The model under review builds one solid part; all positions refer to its coordinate system, in mm. A direction names the side the tool comes from. Give positions to 0.01 mm unless a question says otherwise; leave off trailing zeros. Order: outer loops, then holes, each group sorted by start corner. A loop starts at its lowest first (then second) coordinate and runs counter-clockwise, first axis right, second up. Notation, with made-up numbers: (-16.75, 77.5) - (25.25, 77.5) arc R30 ccw to (25.25, 116.5) - close; hole circle Ø3 at (4, 29.25). An arc over 180 degrees is marked (long way). Use a Markdown table: item, result. Add a question column.
```python
from build123d import *

# Parameters (mm, degrees)
F1_DEPTH  = 12.7
F2_R      = 7.5104207728
F3_DEPTH  = 12.701
F4_W      = 187.1625185013
F4_H      = 16.4809370326
F4_W_2    = 34.8658077419
F4_H_2    = 35.9553694725
F5_DEPTH  = 12.7
F5_FACE_R = 7.5104207728
F5_FACE_W = 34.8658077419
F5_FACE_H = 35.9553694725
F6_DEPTH  = 25.4
F7_DEPTH  = 12.7
F9_DEPTH  = 38.354


with BuildPart() as f1:
    # F0 (on Top) → F1 (new body)
    with BuildSketch(Plane.XY):
        Polygon((21.6443181937, 44.9448898435), (-21.6443181937, 44.9448898435), (-48.6343415176, 11.1004710827), (-39.001713719, -31.1028288117), (0, -49.8850642288), (39.001713719, -31.1028288117), (48.6343415176, 11.1004710827), align=None)
    extrude(amount=F1_DEPTH)

    # F2 (on face) → F3 (cut, through all)
    with BuildSketch(Plane.XY.offset(12.7)):
        with Locations((-21.6443181937, 11.1004710827)):
            Circle(F2_R)
        with Locations((21.6443181937, 11.1004710827)):
            Circle(F2_R)
        with BuildLine():
            ThreePointArc((-22.3923972439, -17.5961239861), (-20.1468702335, -19.4861496183), (-17.2912654826, -20.1644636691))
            Line((-17.2912654826, -20.1644636691), (19.5472728087, -20.1644636691))
            ThreePointArc((19.5472728087, -20.1644636691), (21.5385429204, -19.8441687483), (23.3289331258, -18.9155954304))
            Line((23.3289331258, -18.9155954304), (29.0724616498, -14.657702297))
            Line((29.0724616498, -14.657702297), (-24.5707594616, -14.657702297))
            Line((-24.5707594616, -14.657702297), (-22.3923972439, -17.5961239861))
        make_face()
    extrude(amount=-F3_DEPTH, mode=Mode.SUBTRACT)

    # F4 (on face) → F5 (join)
    with BuildSketch(Plane.XY.offset(12.7)):
        with BuildLine():
            Line((56.5410580551, -83.4953508641), (19.5008568595, -74.5715907042))
            Line((19.5008568595, -74.5715907042), (-19.5008568595, -74.5715907042))
            Line((-19.5008568595, -74.5715907042), (-56.5410580551, -83.4953508641))
            add(Edge.make_bspline(
                [(-56.5410580551, -83.4953508641), (-37.4583826818, -107.754176934), (0, -155.2743553327), (37.4583826818, -107.754176934), (56.5410580551, -83.4953508641)],
                knots=[0, 0, 0, 0, 0.5, 1, 1, 1, 1], degree=3))
        make_face()
        with BuildLine():
            Line((93.5812592506, -92.419111024), (56.5410580551, -83.4953508641))
            add(Edge.make_bspline(
                [(-56.5410580551, -83.4953508641), (-37.4583826818, -107.754176934), (0, -155.2743553327), (37.4583826818, -107.754176934), (56.5410580551, -83.4953508641)],
                knots=[0, 0, 0, 0, 0.5, 1, 1, 1, 1], degree=3))
            Line((-56.5410580551, -83.4953508641), (-93.5812592506, -92.419111024))
            Line((-93.5812592506, -92.419111024), (-93.5812592506, -135.6894243062))
            Line((-93.5812592506, -135.6894243062), (-93.5812592506, -239.1290962696))
            Line((-93.5812592506, -239.1290962696), (93.5812592506, -239.1290962696))
            Line((93.5812592506, -239.1290962696), (93.5812592506, -135.6894243062))
            Line((93.5812592506, -135.6894243062), (93.5812592506, -92.419111024))
        make_face()
        with BuildLine():
            Line((192.9354845729, -199.789452925), (93.5812592506, -92.419111024))
            Line((93.5812592506, -92.419111024), (93.5812592506, -135.6894243062))
            Line((93.5812592506, -135.6894243062), (171.3652932207, -219.7492445575))
            ThreePointArc((171.3652932207, -219.7492445575), (193.3684597033, -221.8925180787), (192.9354845729, -199.789452925))
        make_face()
        with BuildLine():
            Line((-93.5812592506, -135.6894243062), (-93.5812592506, -92.419111024))
            Line((-93.5812592506, -92.419111024), (-192.9354845729, -199.789452925))
            ThreePointArc((-192.9354845729, -199.789452925), (-193.3684597033, -221.8925180787), (-171.3652932207, -219.7492445575))
            Line((-171.3652932207, -219.7492445575), (-93.5812592506, -135.6894243062))
        make_face()
        with Locations((0, -247.3695647859)):
            Rectangle(F4_W, F4_H)
        Polygon((93.5812592506, -410.4407429695), (93.5812592506, -255.6100333022), (-93.5812592506, -255.6100333022), (-93.5812592506, -410.4407429695), (-67.6731318235, -410.4407429695), (-32.8073054552, -410.4407429695), (0, -410.4407429695), (32.8073054552, -410.4407429695), (67.6731318235, -410.4407429695), align=None)
        with Locations((57.6258767396, -294.4029867649)):
            Rectangle(F4_W_2, F4_H_2, mode=Mode.SUBTRACT)
        with BuildLine():
            Line((67.6731318235, -537.919596071), (67.6731318235, -410.4407429695))
            Line((67.6731318235, -410.4407429695), (32.8073054552, -410.4407429695))
            Line((32.8073054552, -410.4407429695), (32.8073054552, -537.919596071))
            ThreePointArc((32.8073054552, -537.919596071), (50.2402186394, -556.4753226857), (67.6731318235, -537.919596071))
        make_face()
        with BuildLine():
            Line((-32.8073054552, -410.4407429695), (-67.6731318235, -410.4407429695))
            Line((-67.6731318235, -410.4407429695), (-67.6731318235, -537.919596071))
            ThreePointArc((-67.6731318235, -537.919596071), (-50.2402186394, -556.4753226857), (-32.8073054552, -537.919596071))
            Line((-32.8073054552, -537.919596071), (-32.8073054552, -410.4407429695))
        make_face()
        Polygon((0, -49.8850642288), (-19.5008568595, -40.4939465203), (-19.5008568595, -74.5715907042), (19.5008568595, -74.5715907042), (19.5008568595, -40.4939465203), align=None)
    extrude(amount=-F5_DEPTH)

    # F4 (on face) + F5_face (on face) → F6 (join)
    with BuildSketch(Plane.XY.offset(12.7)):
        with BuildLine():
            Line((56.5410580551, -83.4953508641), (19.5008568595, -74.5715907042))
            Line((19.5008568595, -74.5715907042), (-19.5008568595, -74.5715907042))
            Line((-19.5008568595, -74.5715907042), (-56.5410580551, -83.4953508641))
            add(Edge.make_bspline(
                [(-56.5410580551, -83.4953508641), (-37.4583826818, -107.754176934), (0, -155.2743553327), (37.4583826818, -107.754176934), (56.5410580551, -83.4953508641)],
                knots=[0, 0, 0, 0, 0.5, 1, 1, 1, 1], degree=3))
        make_face()
        with BuildLine():
            Line((93.5812592506, -92.419111024), (56.5410580551, -83.4953508641))
            add(Edge.make_bspline(
                [(-56.5410580551, -83.4953508641), (-37.4583826818, -107.754176934), (0, -155.2743553327), (37.4583826818, -107.754176934), (56.5410580551, -83.4953508641)],
                knots=[0, 0, 0, 0, 0.5, 1, 1, 1, 1], degree=3))
            Line((-56.5410580551, -83.4953508641), (-93.5812592506, -92.419111024))
            Line((-93.5812592506, -92.419111024), (-93.5812592506, -135.6894243062))
            Line((-93.5812592506, -135.6894243062), (-93.5812592506, -239.1290962696))
            Line((-93.5812592506, -239.1290962696), (93.5812592506, -239.1290962696))
            Line((93.5812592506, -239.1290962696), (93.5812592506, -135.6894243062))
            Line((93.5812592506, -135.6894243062), (93.5812592506, -92.419111024))
        make_face()
        with BuildLine():
            Line((192.9354845729, -199.789452925), (93.5812592506, -92.419111024))
            Line((93.5812592506, -92.419111024), (93.5812592506, -135.6894243062))
            Line((93.5812592506, -135.6894243062), (171.3652932207, -219.7492445575))
            ThreePointArc((171.3652932207, -219.7492445575), (193.3684597033, -221.8925180787), (192.9354845729, -199.789452925))
        make_face()
        with BuildLine():
            Line((-93.5812592506, -135.6894243062), (-93.5812592506, -92.419111024))
            Line((-93.5812592506, -92.419111024), (-192.9354845729, -199.789452925))
            ThreePointArc((-192.9354845729, -199.789452925), (-193.3684597033, -221.8925180787), (-171.3652932207, -219.7492445575))
            Line((-171.3652932207, -219.7492445575), (-93.5812592506, -135.6894243062))
        make_face()
        with Locations((0, -247.3695647859)):
            Rectangle(F4_W, F4_H)
        Polygon((93.5812592506, -410.4407429695), (93.5812592506, -255.6100333022), (-93.5812592506, -255.6100333022), (-93.5812592506, -410.4407429695), (-67.6731318235, -410.4407429695), (-32.8073054552, -410.4407429695), (0, -410.4407429695), (32.8073054552, -410.4407429695), (67.6731318235, -410.4407429695), align=None)
        with Locations((57.6258767396, -294.4029867649)):
            Rectangle(F4_W_2, F4_H_2, mode=Mode.SUBTRACT)
        with BuildLine():
            Line((67.6731318235, -537.919596071), (67.6731318235, -410.4407429695))
            Line((67.6731318235, -410.4407429695), (32.8073054552, -410.4407429695))
            Line((32.8073054552, -410.4407429695), (32.8073054552, -537.919596071))
            ThreePointArc((32.8073054552, -537.919596071), (50.2402186394, -556.4753226857), (67.6731318235, -537.919596071))
        make_face()
        with BuildLine():
            Line((-32.8073054552, -410.4407429695), (-67.6731318235, -410.4407429695))
            Line((-67.6731318235, -410.4407429695), (-67.6731318235, -537.919596071))
            ThreePointArc((-67.6731318235, -537.919596071), (-50.2402186394, -556.4753226857), (-32.8073054552, -537.919596071))
            Line((-32.8073054552, -537.919596071), (-32.8073054552, -410.4407429695))
        make_face()
    with BuildSketch(Plane(origin=(-0.8446468995, -244.4359717848, 12.7), x_dir=(1, 0, 0), z_dir=(0, 0, 1))):
        with BuildLine():
            Line((22.4889650932, 289.3808616283), (-20.7996712942, 289.3808616283))
            Line((-20.7996712942, 289.3808616283), (-47.7896946182, 255.5364428675))
            Line((-47.7896946182, 255.5364428675), (-38.1570668195, 213.3331429731))
            Line((-38.1570668195, 213.3331429731), (-18.65620996, 203.9420252645))
            Line((-18.65620996, 203.9420252645), (-18.65620996, 169.8643810806))
            Line((-18.65620996, 169.8643810806), (-92.7366123512, 152.0168607608))
            Line((-92.7366123512, 152.0168607608), (-192.0908376734, 44.6465188598))
            ThreePointArc((-192.0908376734, 44.6465188598), (-192.5238128038, 22.5434537061), (-170.5206463212, 24.6867272273))
            Line((-170.5206463212, 24.6867272273), (-92.7366123512, 108.7465474786))
            Line((-92.7366123512, 108.7465474786), (-92.7366123512, -166.0047711847))
            Line((-92.7366123512, -166.0047711847), (-66.8284849241, -166.0047711847))
            Line((-66.8284849241, -166.0047711847), (-66.8284849241, -293.4836242862))
            ThreePointArc((-66.8284849241, -293.4836242862), (-49.3955717399, -312.0393509009), (-31.9626585557, -293.4836242862))
            Line((-31.9626585557, -293.4836242862), (-31.9626585557, -166.0047711847))
            Line((-31.9626585557, -166.0047711847), (33.6519523547, -166.0047711847))
            Line((33.6519523547, -166.0047711847), (33.6519523547, -293.4836242862))
            ThreePointArc((33.6519523547, -293.4836242862), (51.0848655389, -312.0393509009), (68.517778723, -293.4836242862))
            Line((68.517778723, -293.4836242862), (68.517778723, -166.0047711847))
            Line((68.517778723, -166.0047711847), (94.4259061501, -166.0047711847))
            Line((94.4259061501, -166.0047711847), (94.4259061501, 108.7465474786))
            Line((94.4259061501, 108.7465474786), (172.2099401201, 24.6867272273))
            ThreePointArc((172.2099401201, 24.6867272273), (194.2131066028, 22.5434537061), (193.7801314724, 44.6465188598))
            Line((193.7801314724, 44.6465188598), (94.4259061501, 152.0168607608))
            Line((94.4259061501, 152.0168607608), (20.345503759, 169.8643810806))
            Line((20.345503759, 169.8643810806), (20.345503759, 203.9420252645))
            Line((20.345503759, 203.9420252645), (39.8463606185, 213.3331429731))
            Line((39.8463606185, 213.3331429731), (49.4789884171, 255.5364428675))
            Line((49.4789884171, 255.5364428675), (22.4889650932, 289.3808616283))
        make_face()
        with BuildLine():
            Line((-21.5477503444, 226.8398477987), (-23.7261125621, 229.7782694878))
            Line((-23.7261125621, 229.7782694878), (29.9171085493, 229.7782694878))
            Line((29.9171085493, 229.7782694878), (24.1735800252, 225.5203763544))
            ThreePointArc((24.1735800252, 225.5203763544), (22.3831898199, 224.5918030365), (20.3919197082, 224.2715081157))
            Line((20.3919197082, 224.2715081157), (-16.4466185831, 224.2715081157))
            ThreePointArc((-16.4466185831, 224.2715081157), (-19.302223334, 224.9498221665), (-21.5477503444, 226.8398477987))
        make_face(mode=Mode.SUBTRACT)
        with Locations((-20.7996712942, 255.5364428675)):
            Circle(F5_FACE_R, mode=Mode.SUBTRACT)
        with Locations((22.4889650932, 255.5364428675)):
            Circle(F5_FACE_R, mode=Mode.SUBTRACT)
        with Locations((58.4705236391, -49.9670149801)):
            Rectangle(F5_FACE_W, F5_FACE_H, mode=Mode.SUBTRACT)
    extrude(amount=F6_DEPTH)

    # F4 (on face) → F7 (cut)
    with BuildSketch(Plane.XY.offset(12.7)):
        with Locations((0, -247.3695647859)):
            Rectangle(F4_W, F4_H)
    extrude(amount=-F7_DEPTH, mode=Mode.SUBTRACT)

    # F8 (on face) → F9 (join)
    with BuildSketch(Plane(origin=(0, 0, 0), x_dir=(1, 0, 0), z_dir=(0, 0, -1))):
        Polygon((21.6443181937, -104.6233549714), (21.6443181937, -44.9448898435), (-21.6443181937, -44.9448898435), (-21.6443181937, -104.6233549714), (0, -119.0398335457), align=None)
    extrude(amount=-F9_DEPTH)


solid = f1.part
```
Q1. We need section B-B (z = 23.5). Count the separate pieces of the cut face and the enclosed holes in it, plus the area to 3 significant figures.
Q2. Clearance check with flat-ended pins moving along their axes: P1, Ø8, axis at x = 43, y = -244.5, coming from the -Z side; P2, Ø6.5, axis at x = 13, z = 7.5, coming from the -Y side; P3, Ø1.5, axis at y = -267, z = 32.5, coming from the +X side. State where each tip first meets the part, or that it passes through.
Q3. We need section D-D (x = 81.5). Write out the cut boundary in (y, z), plus the area to 3 significant figures.
Q4. Machinability: for faces 1 (the flat face through (-21.644, 74, 19)), 2 (the flat face through (80, -410.441, 19)), 3 (the flat face through (-67.673, -473, 19)), 4 (the flat face through (19.501, -58, 19)), 5 (the flat face through (32.807, -473, 19)), which of the approach directions +Z, -Z, +X, -X, +Y, -Y give a long, thin tool a straight path to every point of the face, cutting with its end or side? Answer none if there is none.
Q5. Wall thickness on probe 1 along Y at (x, z) = (-27, 14.5); probe 2 along X at (y, z) = (-504.5, 33.5); probe 3 along X at (y, z) = (-224, 5.5): over which ranges is each line inside the solid? List them lowest first.
Q6. We need section C-C (y = -355). Write out the cut boundary in (x, z).
Q7. Draft analysis for pull direction X (two halves, no side actions). For faces 6 (the flat face through (-93.581, -271, 19)), 7 (the flat face through (0, 81, 38.354)), 8 (the cylindrical face through (-50.64, -556.47, 18.78)), 9 (the flat face through (-19.501, -57, 19)), state which applies: pulls with the +X half, pulls with the -X half, needs draft (parallel to the pull), parting line crosses it, or undercut.
Q8. We need section A-A (y = -453). Write out the cut boundary in (x, z), plus the area to 3 significant figures.
Here are the results:
| question | item | result |
|---|---|---|
| 1 | separate pieces | 1 |
| 1 | enclosed holes | 4 |
| 1 | area | 88,900 mm2 |
| 2 | P1 | z = 12.7 |
| 2 | P2 | y = -410.44 |
| 2 | P3 | x = 93.58 |
| 3 | outline | (-410.44, 0) - (-255.61, 0) - (-255.61, 12.7) - (-239.13, 12.7) - (-239.13, 0) - (-89.51, 0) - (-89.51, 38.1) - (-410.44, 38.1) - close |
| 3 | area | 12,000 mm2 |
| 4 | face 1 | +Z, -Z, -X, +Y |
| 4 | face 2 | +Z, -Z, +X, -Y |
| 4 | face 3 | +Z, -Z, -X, -Y |
| 4 | face 4 | +Z, -Z, +X |
| 4 | face 5 | +Z, -Z, -Y |
| 5 | probe 1 | -410.44 to -76.38, -36.88 to 5.84, 16.37 to 38.23 |
| 5 | probe 2 | -67.67 to -32.81, 32.81 to 67.67 |
| 5 | probe 3 | -190.44 to -176.2, -93.58 to 93.58, 176.2 to 190.44 |
| 6 | outline | (-93.58, 0) - (93.58, 0) - (93.58, 38.1) - (-93.58, 38.1) - close |
| 7 | face 6 | undercut |
| 7 | face 7 | needs draft |
| 7 | face 8 | undercut |
| 7 | face 9 | pulls with the -X half |
| 8 | outline | (-67.67, 0) - (-32.81, 0) - (-32.81, 38.1) - (-67.67, 38.1) - close; (32.81, 0) - (67.67, 0) - (67.67, 38.1) - (32.81, 38.1) - close |
| 8 | area | 2,660 mm2 |
